CAD build for the part. Positions are in the model's coordinates, mm. A direction names the side the tool comes from. Coordinates: 2 decimals unless noted, no trailing zeros. Order: outer loops, then holes, each group sorted by start corner. A loop starts at its lowest first (then second) coordinate and runs counter-clockwise, first axis right, second up. Notation, with made-up numbers: (-2, 1) -> (31, 1) arc R24 cw to (31, 24) -> close; hole circle Ø3 at (81.5, 79). An arc over 180 degrees is marked (long way). Use one line per item in the form item = value. Start each with the question number.
from build123d import *

# Parameters (mm, degrees)
SKETCH1_R           = 11
SKETCH1_R_2         = 6
SKETCH1_R_3         = 7.5
SKETCH1_R_4         = 2.1
SKETCH1_R_5         = 19
SKETCH1_R_6         = 2.5
BOSS_EXTRUDE1_DEPTH = 5
SKETCH6_R           = 4
BOSS_EXTRUDE2_DEPTH = 5
FILLET1_R           = 10
FILLET2_R           = 40
CUT_EXTRUDE5_DEPTH  = 159.977801764
SKETCH9_R           = 4
BOSS_EXTRUDE3_DEPTH = 5
FILLET4_R           = 25
FILLET6_R           = 40
FILLET7_R           = 12


with BuildPart() as part:
    # Sketch1 → Boss-Extrude1 (new body)
    with BuildSketch(Plane(origin=(0, 0, 0), x_dir=(1, 0, 0), z_dir=(0, 1, 0))):
        with BuildLine():
            Line((-97.5, 40), (97.5, 40))
            ThreePointArc((97.5, 40), (137.5, 0), (97.5, -40))
            Line((97.5, -40), (-97.5, -40))
            ThreePointArc((-97.5, -40), (-137.5, 0), (-97.5, 40))
        make_face()
        with Locations(Location((97.5, 0, 0), (0, 0, 270))):
            Circle(SKETCH1_R, mode=Mode.SUBTRACT)
        with Locations(Location((35.8, 0, 0), (0, 0, 270))):
            Circle(SKETCH1_R_2, mode=Mode.SUBTRACT)
        with Locations(Location((-97.5, 0, 0), (0, 0, 270))):
            Circle(SKETCH1_R_3, mode=Mode.SUBTRACT)
        with Locations(Location((-97.5, -20, 0), (0, 0, 270))):
            Circle(SKETCH1_R_4, mode=Mode.SUBTRACT)
        with Locations(Location((-117.5, 0, 0), (0, 0, 270))):
            Circle(SKETCH1_R_4, mode=Mode.SUBTRACT)
        with Locations(Location((-97.5, 20, 0), (0, 0, 270))):
            Circle(SKETCH1_R_4, mode=Mode.SUBTRACT)
        with Locations(Location((-77.5, 0, 0), (0, 0, 270))):
            Circle(SKETCH1_R_4, mode=Mode.SUBTRACT)
        with Locations(Location((-25.9, 0, 0), (0, 0, 270))):
            Circle(SKETCH1_R_5, mode=Mode.SUBTRACT)
        with Locations(Location((-27.5, 35, 0), (0, 0, 270))):
            Circle(SKETCH1_R_4, mode=Mode.SUBTRACT)
        with Locations(Location((37.5, 35, 0), (0, 0, 270))):
            Circle(SKETCH1_R_4, mode=Mode.SUBTRACT)
        with Locations(Location((52.5, -35, 0), (0, 0, 270))):
            Circle(SKETCH1_R_4, mode=Mode.SUBTRACT)
        with Locations(Location((-27.5, -35, 0), (0, 0, 270))):
            Circle(SKETCH1_R_4, mode=Mode.SUBTRACT)
        with Locations(Location((115, 17.5, 0), (0, 0, 270))):
            Circle(SKETCH1_R_4, mode=Mode.SUBTRACT)
        with Locations(Location((115, -17.5, 0), (0, 0, 270))):
            Circle(SKETCH1_R_4, mode=Mode.SUBTRACT)
        with Locations(Location((80, -17.5, 0), (0, 0, 270))):
            Circle(SKETCH1_R_4, mode=Mode.SUBTRACT)
        with Locations(Location((80, 17.5, 0), (0, 0, 270))):
            Circle(SKETCH1_R_4, mode=Mode.SUBTRACT)
        with Locations(Location((-2.33, -23.57, 0), (0, 0, 270))):
            Circle(SKETCH1_R_4, mode=Mode.SUBTRACT)
        with Locations(Location((-49.47, -23.57, 0), (0, 0, 270))):
            Circle(SKETCH1_R_4, mode=Mode.SUBTRACT)
        with Locations(Location((-49.47, 23.57, 0), (0, 0, 270))):
            Circle(SKETCH1_R_4, mode=Mode.SUBTRACT)
        with Locations(Location((-2.33, 23.57, 0), (0, 0, 270))):
            Circle(SKETCH1_R_4, mode=Mode.SUBTRACT)
        with Locations(Location((55.8, 0, 0), (0, 0, 270))):
            Circle(SKETCH1_R_4, mode=Mode.SUBTRACT)
        with Locations(Location((35.8, -20, 0), (0, 0, 270))):
            Circle(SKETCH1_R_4, mode=Mode.SUBTRACT)
        with Locations(Location((15.8, 0, 0), (0, 0, 270))):
            Circle(SKETCH1_R_4, mode=Mode.SUBTRACT)
        with Locations(Location((35.8, 20, 0), (0, 0, 270))):
            Circle(SKETCH1_R_4, mode=Mode.SUBTRACT)
        with Locations(Location((61.5, -30, 0), (0, 0, 270))):
            Circle(SKETCH1_R_6, mode=Mode.SUBTRACT)
    extrude(amount=BOSS_EXTRUDE1_DEPTH)

    # Sketch6 → Boss-Extrude2 (add)
    with BuildSketch(Plane(origin=(0, 5, 0), x_dir=(1, 0, 0), z_dir=(0, 1, 0))):
        Polygon((-52.5, 40), (-77.5, 83.301270189), (-96.25, 72.475952642), (-77.5, 40), align=None)
        with Locations(Location((-80.857695155, 69.815698604, 0), (0, 0, 270))):
            Circle(SKETCH6_R, mode=Mode.SUBTRACT)
    extrude(amount=-BOSS_EXTRUDE2_DEPTH)

    # Fillet1
    fillet1_edges = [part.edges().sort_by_distance(p)[0] for p in [
        (-77.5, 2.5, -40),
        (-96.25, 2.5, -72.475952642),
        (-77.5, 2.5, -83.301270189),
    ]]
    fillet(fillet1_edges, radius=FILLET1_R)

    # Fillet2
    fillet2_edges = [part.edges().sort_by_distance(p)[0] for p in [
        (-52.5, 2.5, -40),
    ]]
    fillet(fillet2_edges, radius=FILLET2_R)

    # Sketch8 → Cut-Extrude5 (cut, through all)
    with BuildSketch(Plane(origin=(0, 5, 0), x_dir=(1, 0, 0), z_dir=(0, 1, 0))):
        with BuildLine():
            Line((60.263644342, 18.045663623), (61.309513255, 30))
            ThreePointArc((61.309513255, 30), (64.017889357, 32.272597388), (66.290486745, 29.564221286))
            Line((66.290486745, 29.564221286), (65.244617832, 17.609884909))
            ThreePointArc((65.244617832, 17.609884909), (62.53624173, 15.337287521), (60.263644342, 18.045663623))
        make_face()
    extrude(amount=-CUT_EXTRUDE5_DEPTH, mode=Mode.SUBTRACT)

    # Sketch9 → Boss-Extrude3 (add)
    with BuildSketch(Plane(origin=(0, 5, 0), x_dir=(1, 0, 0), z_dir=(0, 1, 0))):
        Polygon((17.5, 40), (42.5, 40), (70.24867186, 81.593403443), (47.5, 91.961524227), align=None)
        with Locations(Location((53.850852961, 76.961524227, 0), (0, 0, 270))):
            Circle(SKETCH9_R, mode=Mode.SUBTRACT)
    extrude(amount=-BOSS_EXTRUDE3_DEPTH)

    # Fillet4
    fillet4_edges = [part.edges().sort_by_distance(p)[0] for p in [
        (42.5, 2.5, -40),
    ]]
    fillet(fillet4_edges, radius=FILLET4_R)

    # Fillet6
    fillet6_edges = [part.edges().sort_by_distance(p)[0] for p in [
        (17.5, 2.5, -40),
    ]]
    fillet(fillet6_edges, radius=FILLET6_R)

    # Fillet7
    fillet7_edges = [part.edges().sort_by_distance(p)[0] for p in [
        (47.5, 2.5, -91.961524227),
        (70.24867186, 2.5, -81.593403443),
    ]]
    fillet(fillet7_edges, radius=FILLET7_R)


solid = part.part
1) Cut at D-D on x = 22. Give the cut face in (y, z).
2) Cut at A-A on x = 100. Give the cut face in (y, z), then the cut area to 3 significant figures.
3) Two-plate mould, pull along X, no slides. Class faces 5 (the face through (-42.756, 2.465, 8.767)), 6 (the face through (69.32, 2.46, -49.88)), 7 (the face through (-92.277, 2.465, -71.298)): released by +X, released by -X, zero draft, split by the parting line, or undercut.
4) Cut at C-C on y = 3.2. Count the separate pieces of the cut face and the enclosed holes in it, then the cut area to 3 significant figures.
5) Drop flat-ended pins along their axis: P1, Ø3, axis at y = 3.5, z = -74.5, coming from the +X side (3 decimals); P2, Ø3, axis at x = 22, y = 2, coming from the -Z side; P3, Ø3, axis at y = 1, z = -17.5, coming from the -X side; P4, Ø7, axis at x = 53.85, z = -76.96, coming from the -Y side. Give the stop position or say it passes through.
6) Probe L1, parallel to X at y = 1.3, z = -35; L2, parallel to Z at x = -48, y = 2.85; L3, parallel to X at y = 1.3, z = -45.5. List the from-to ranges inside material, lowest first.
7) Cut at B-B on z = 30. Give the cut face in (x, y), then the cut area to 3 significant figures.
8) 3-axis set-ups, long thin cutter, end or side, ignore diameter. For faces 1 (the face through (-88.74, 2.54, -59.47)), 2 (the face through (2, 5, -11)), 3 (the face through (65.775, 2.535, -23.671)), 4 (the face through (-49.152, 2.465, -45.213)): which of +Z, -Z, +X, -X, +Y, -Y reach the whole face in a straight line?
Values follow:
q1.outline = (0, -51.04) -> (5, -51.04) -> (5, 40) -> (0, 40) -> close
q2.outline = (0, -39.92) -> (5, -39.92) -> (5, -10.71) -> (0, -10.71) -> close; (0, 10.71) -> (5, 10.71) -> (5, 39.92) -> (0, 39.92) -> close
q2.area = 292 mm^2
q3.face_5 = undercut
q3.face_6 = released by +X
q3.face_7 = released by -X
q4.separate_pieces = 1
q4.enclosed_holes = 28
q4.area = 21,200 mm^2
q5.P1 = 65.865
q5.P2 = -52.55
q5.P3 = -134.16
q5.P4 = through
q6.L1 = -116.86 to -29.6, -25.4 to 35.4, 39.6 to 116.86
q6.L2 = -44.58 to -25.07, -22.07 to 22.07, 25.07 to 40
q6.L3 = -85.89 to -49.65, 14.65 to 73.59
q7.outline = (-123.96, 0) -> (59, 0) -> (59, 5) -> (-123.96, 5) -> close; (64, 0) -> (123.96, 0) -> (123.96, 5) -> (64, 5) -> close
q7.area = 1,210 mm^2
q8.face_1 = -X, +Y, -Y
q8.face_2 = +Z, -Z, +X, -X, +Y
q8.face_3 = +Y, -Y
q8.face_4 = -Z, +Y, -Y
